Part print with two shaded views. Sizes in mm from the minimum x, y, z corner. A direction names the side the tool comes from. Coordinates: 2 decimals unless noted, no trailing zeros. Loops run counter-clockwise (first coordinate to the right, second up) from the corner with the lowest first, then second, coordinate; pieces in that order, holes last. Notation, with made-up numbers: (29, 81.5) -> (33, 81.5) arc R23 cw to (33, 115.5) -> close; hole circle Ø5 at (-8.5, -22). An arc over 180 degrees is marked (long way). Return JSON: item names as keys, results as strings. Group by question number.
(1) Probe L1, parallel to X at y = 13.5, z = 4; L2, parallel to Y at x = 5, z = 0.5; L3, parallel to Y at x = 21.5, z = 5.25. List the from-to ranges inside material, lowest first.
(2) Saw through at D-D on x = 39.5. Write the cut outline in (y, z), then the cut area to 3 significant figures.
(3) Flat gauge pins, fed straight in: pin 1 Ø3 at (x, z) = (8, 3.5) entering from +Y; pin 2 Ø3 at (y, z) = (13, 1.5) entering from -X. Where does each tip first touch, or does it go through?
(4) Tool access for the marked faces 1, 2 and 3: list every direction of +Z, -Z, +X, -X, +Y, -Y with a clear straight run to the whole face (end or side of a thin tool).
(5) Saw through at B-B on z = 4.5. Write the cut outline in (x, y).
(6) Saw through at C-C on y = 12. Write the cut outline in (x, z), then the cut area to 3 significant figures.
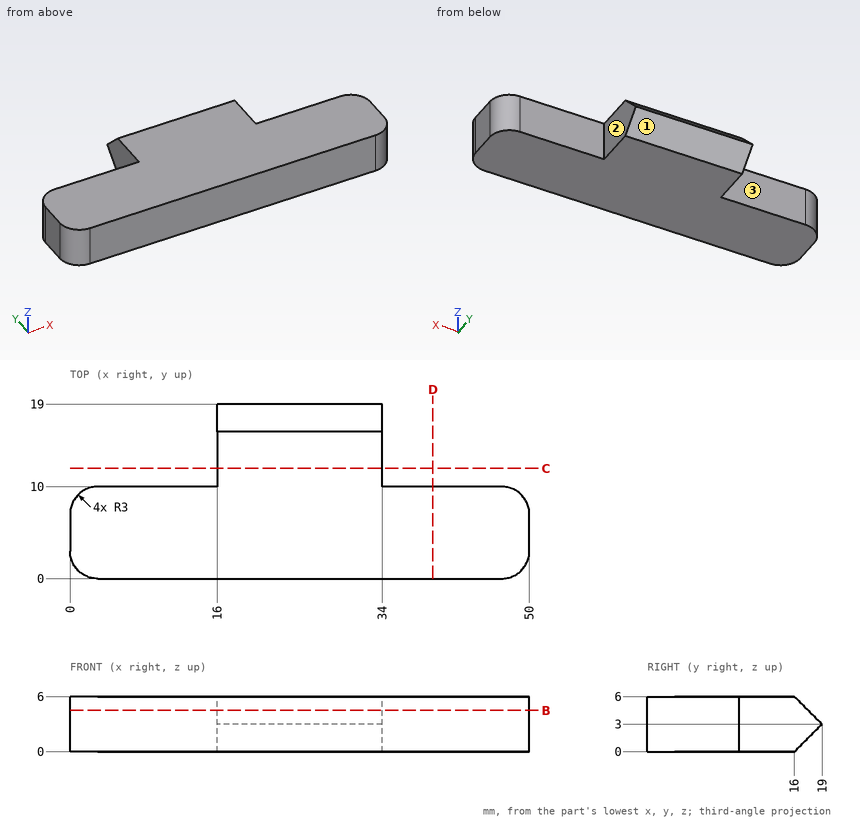
Geometry results:
{
 "1": {"L1": "16 to 34", "L2": "0 to 10", "L3": "0 to 16.75"},
 "2": {"outline": "(0, 0) -> (10, 0) -> (10, 6) -> (0, 6) -> close", "area": "60.0 mm²"},
 "3": {"pin 1": "y = 10", "pin 2": "x = 16"},
 "4": {"face 1": "-Z, +X, -X, +Y", "face 2": "+Z, -Z, +X, +Y", "face 3": "+Z, -Z, -X, +Y"},
 "5": {"outline": "(0, 3) arc R3 ccw to (3, 0) -> (47, 0) arc R3 ccw to (50, 3) -> (50, 7) arc R3 ccw to (47, 10) -> (34, 10) -> (34, 17.5) -> (16, 17.5) -> (16, 10) -> (3, 10) arc R3 ccw to (0, 7) -> close"},
 "6": {"outline": "(16, 0) -> (34, 0) -> (34, 6) -> (16, 6) -> close", "area": "108 mm²"}
}
